Verification items for this drawing (mm, ordinates from the low corner). A direction names the side the tool comes from. Give positions to 0.01 mm unless a question says otherwise; leave off trailing zeros. Write each loop counter-clockwise with the first axis right and the second up, starting at its lowest first coordinate (ties: lowest second). Pieces come first, ordered by that corner, then holes. Notation, with made-up numbers: (22, 29.25) -> (28, 29.25) arc R14 cw to (28, 37.25) -> close; hole circle Ø7 at (66, -2). An arc over 180 degrees is marked (long way). Answer as a JSON object with one key per item and string values.
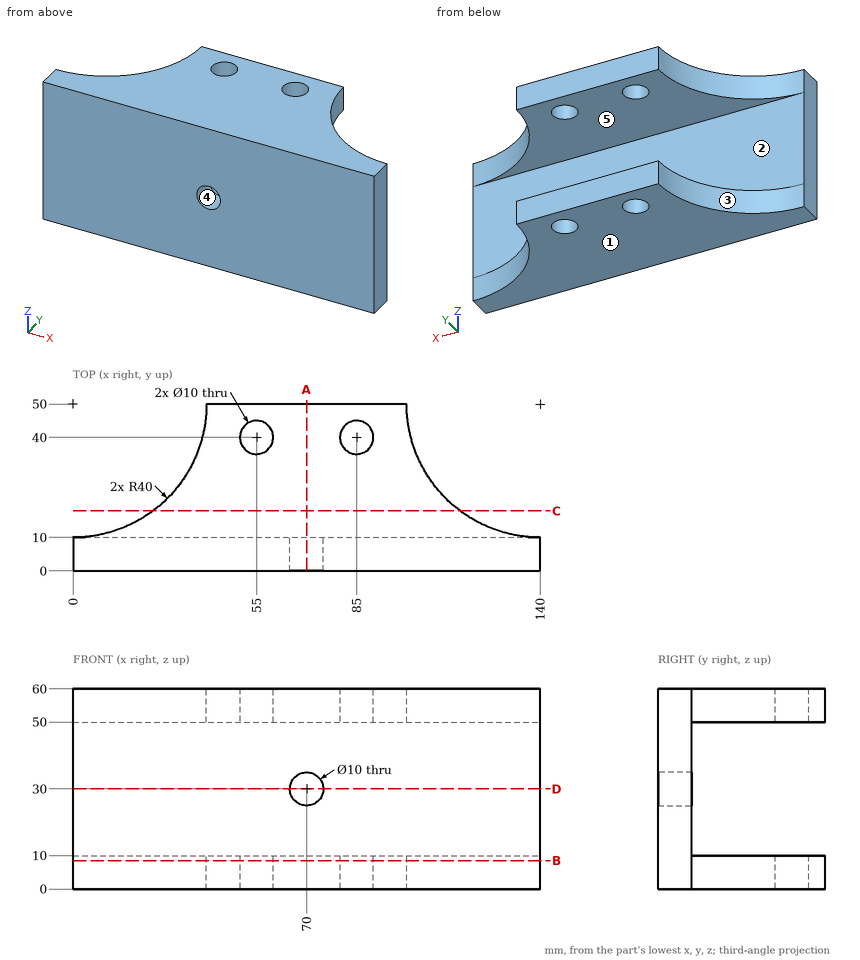
1. Mould release check, pull along Z, two halves, no side actions. Record for the marked faces 1, 2 and 3: released by +Z, released by -Z, zero draft, split by the parting line, or undercut.
Determined:
{"face 1": "released by -Z", "face 2": "undercut", "face 3": "zero draft"}
2. Sectioned sample at C-C, the plane y = 18. Enter the section's corners in (x, z).
Determined:
{"outline": "(24, 0) -> (116, 0) -> (116, 10) -> (24, 10) -> close; (24, 50) -> (116, 50) -> (116, 60) -> (24, 60) -> close"}
3. Sectioned sample at B-B, the plane z = 8.5. Enter the section's corners in (x, y).
Determined:
{"outline": "(0, 0) -> (140, 0) -> (140, 10) arc R40 cw to (100, 50) -> (40, 50) arc R40 cw to (0, 10) -> close; hole circle Ø10 at (55, 40); hole circle Ø10 at (85, 40)"}
4. Sectioned sample at A-A, the plane x = 70. Enter the section's corners in (y, z).
Determined:
{"outline": "(0, 0) -> (50, 0) -> (50, 10) -> (10, 10) -> (10, 25) -> (0, 25) -> close; (0, 35) -> (10, 35) -> (10, 50) -> (50, 50) -> (50, 60) -> (0, 60) -> close"}
5. Scan lines: L1, parallel to Y at x = 85, z = 56.25; L2, parallel to X at y = 42.5, z = 51.5; L3, parallel to Z at x = 92, y = 11. Record each from-to range of solid material in increasing order. Write a range as [from, to].
Determined:
{"L1": "[0, 35], [45, 50]", "L2": "[39.29, 50.67], [59.33, 80.67], [89.33, 100.71]", "L3": "[0, 10], [50, 60]"}
6. Sectioned sample at D-D, the plane z = 30. Enter the section's corners in (x, y), plus the area to 3 significant figures.
Determined:
{"outline": "(0, 0) -> (65, 0) -> (65, 10) -> (0, 10) -> close; (75, 0) -> (140, 0) -> (140, 10) -> (75, 10) -> close", "area": "1,300 mm^2"}
7. Access from +Z, -Z, +X, -X, +Y, -Y to the whole of each face (thin tool, end or side, straight path). Record for the marked faces 4 and 5.
Determined:
{"face 4": "+Y, -Y", "face 5": "+X, -X, +Y"}
8. Go/stop test with a flat-tipped pin: P1, Ø8, axis at x = 62, z = 17, coming from the +Y side. Record where the tip stops, or that it passes through.
Determined:
{"P1": "y = 10"}
